The model under review builds one solid part; all positions refer to its coordinate system, in mm. Face numbers are marked on the shaded views. A direction names the side the tool comes from. Coordinates: 2 decimals unless noted, no trailing zeros. Loops run counter-clockwise (first coordinate to the right, second up) from the corner with the lowest first, then second, coordinate; pieces in that order, holes last. Notation, with made-up numbers: M 28.5,-9 L 70.5,-9 A14 cw 70.5,1 Z; hole C 22,73 d3. An arc over 180 degrees is marked long. Return JSON: item names as keys, results as strings.
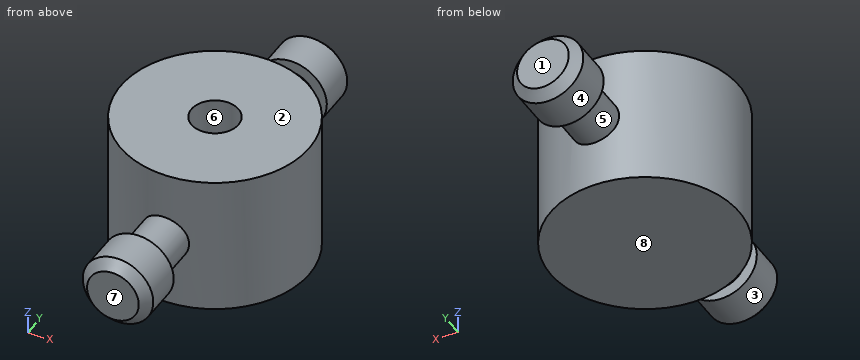
```python
from build123d import *

# Parameters (mm, degrees)
SKETCH1_R                = 20
BOSS_EXTRUDE1_DEPTH      = 30
BOSS_EXTRUDE2_DEPTH      = 30
BOSS_EXTRUDE2_DEPTH_BACK = 30
SKETCH2_R                = 5
SKETCH3_R                = 7.5
BOSS_EXTRUDE3_DEPTH      = 10
CHAMFER1_SIZE            = 2
CHAMFER1_OF_MIRROR1_SIZE = 2
SKETCH4_R                = 5
CUT_EXTRUDE1_DEPTH       = 10


with BuildPart() as part:
    # Sketch1 → Boss-Extrude1 (new body)
    with BuildSketch(Plane.XY):
        Circle(SKETCH1_R)
    extrude(amount=BOSS_EXTRUDE1_DEPTH)

    # Sketch2 → Boss-Extrude2 (add, two sides: drawn at the far end of the back side and taken through both)
    with BuildSketch(Plane(origin=(0, 0, 0), x_dir=(1, 0, 0), z_dir=(0, 1, 0)).offset(-BOSS_EXTRUDE2_DEPTH_BACK)):
        with Locations(Location((0, -15, 0), (0, 0, 270))):
            Circle(SKETCH2_R)
    extrude(amount=BOSS_EXTRUDE2_DEPTH + BOSS_EXTRUDE2_DEPTH_BACK)

    # Sketch3 → Boss-Extrude3 (add)
    with BuildSketch(Plane(origin=(0, 30, 0), x_dir=(1, 0, 0), z_dir=(0, 1, 0))):
        with Locations(Location((0, -15, 0), (0, 0, 270))):
            Circle(SKETCH3_R)
    boss_extrude3 = extrude(amount=BOSS_EXTRUDE3_DEPTH)

    # Chamfer1
    chamfer1_edges = [part.edges().sort_by_distance(p)[0] for p in [
        (0, 40, 7.5),
    ]]
    chamfer(chamfer1_edges, length=CHAMFER1_SIZE)

    # Mirror1: Boss-Extrude3 across plane
    add(boss_extrude3.mirror(Plane.ZX))

    # Chamfer1 of Mirror1
    chamfer1_of_mirror1_edges = [part.edges().sort_by_distance(p)[0] for p in [
        (0, -40, 7.5),
    ]]
    chamfer(chamfer1_of_mirror1_edges, length=CHAMFER1_OF_MIRROR1_SIZE)

    # Sketch4 → Cut-Extrude1 (cut)
    with BuildSketch(Plane.XY.offset(30)):
        Circle(SKETCH4_R)
    extrude(amount=-CUT_EXTRUDE1_DEPTH, mode=Mode.SUBTRACT)


solid = part.part
```
1. Add section B-B on z = 15. Give the boundary of the cut face in (x, y), plus the area to 3 significant figures.
Check values:
{"outline": "M -7.5,-38 L -5.5,-40 L 5.5,-40 L 7.5,-38 L 7.5,-30 L 5,-30 L 5,-19.36 A20 ccw 5,19.36 L 5,30 L 7.5,30 L 7.5,38 L 5.5,40 L -5.5,40 L -7.5,38 L -7.5,30 L -5,30 L -5,19.36 A20 ccw -5,-19.36 L -5,-30 L -7.5,-30 Z", "area": "1,750 mm²"}
2. Insertion check: pin 1 Ø1 at (y, z) = (28.5, 12.5) entering from +X; pin 2 Ø4 at (x, y) = (8, -22) entering from +Z; pin 3 Ø1 at (y, z) = (23.5, 11) entering from -X; pin 4 Ø6 at (x, z) = (-6.5, 7.5) entering from -Y. Each pin has a flat end and moves straight along its axis. Give the tip position at first contact, or say it passes through.
Check values:
{"pin 1": "x = 4.58", "pin 2": "through", "pin 3": "x = -3.57", "pin 4": "y = -38.58"}
3. Add section A-A on x = 0. Give the boundary of the cut face in (y, z).
Check values:
{"outline": "M -40,9.5 L -38,7.5 L -30,7.5 L -30,10 L -20,10 L -20,0 L 20,0 L 20,10 L 30,10 L 30,7.5 L 38,7.5 L 40,9.5 L 40,20.5 L 38,22.5 L 30,22.5 L 30,20 L 20,20 L 20,30 L 5,30 L 5,20 L -5,20 L -5,30 L -20,30 L -20,20 L -30,20 L -30,22.5 L -38,22.5 L -40,20.5 Z"}
4. The part is to be moulded in two halves that separate along Y. For the marked faces 6, 7 and 8, say which applies: released by +Y, released by -Y, zero draft, split by the parting line, or undercut.
Check values:
{"face 6": "undercut", "face 7": "released by -Y", "face 8": "zero draft"}
5. Machinability: for the marked faces 1, 2, 3, 4 and 5, which of the approach directions +Z, -Z, +X, -X, +Y, -Y give a long, thin tool a straight path to every point of the face, cutting with its end or side? Answer none if there is none.
Check values:
{"face 1": "+Z, -Z, +X, -X, +Y", "face 2": "+Z, +X, -X, +Y, -Y", "face 3": "-Y", "face 4": "+Y", "face 5": "none"}
6. Add section C-C on y = 0. Give the boundary of the cut face in (x, z), plus the area to 3 significant figures.
Check values:
{"outline": "M -20,0 L 20,0 L 20,30 L 5,30 L 5,20 L -5,20 L -5,30 L -20,30 Z", "area": "1,100 mm²"}
7. Add section D-D on z = 27. Give the boundary of the cut face in (x, y), plus the area to 3 significant figures.
Check values:
{"outline": "C 0,0 d40; hole C 0,0 d10", "area": "1,180 mm²"}
8. To check wall thickness, follow line 1 (Y direction, x = 0, z = 23.75); line 2 (Z direction, x = 0.5, y = -34); line 3 (X direction, y = -14, z = 26). State the ranges of each line that lie inside material, in increasing order.
Check values:
{"line 1": "-20 to -5, 5 to 20", "line 2": "7.52 to 22.48", "line 3": "-14.28 to 14.28"}
